Input: part model. Units: mm. Frame: model coordinates. A direction names the side the tool comes from. Coordinates: 2 decimals unless noted, no trailing zeros. Loops run counter-clockwise (first coordinate to the right, second up) from the corner with the lowest first, then second, coordinate; pieces in that order, holes last.
Item 1: Ray query, line 1 along Y through (x, z) = (43, 1.4) (3 decimals); line 2 along Y through (x, z) = (12.7, 1.1); line 3 along Y through (x, z) = (63.5, 0.8) (3 decimals). Return the intervals inside material, ascending.
Item 2: Contact query for flat-ended pins moving along their axis: P1, Ø1, axis at x = 19, z = 2, coming from the +Y side; P2, Ø1, axis at y = 23.5, z = 1, coming from the -X side; P3, Ø1, axis at y = -42, z = 2, coming from the -X side; P4, Ø8, axis at x = 77, y = -21, coming from the -Z side. Output: stop coordinate, or through.
Item 3: Section B-B on x = 44. Return loops of the section in (y, z) (3 decimals).
Item 4: Reachability of faces 4 (the flat face through (62, -53.975, 2)), 5 (the cylindrical face through (57.191, 5.716, 1.61)) from +Z, -Z, +X, -X, +Y, -Y: full face, straight path, thin tool, end or side. Return the list, or none.
Item 5: Section A-A on y = 38.1. Return loops of the section in (x, z) (3 decimals), and give its area (3 significant figures).
Item 6: Section D-D on y = 12.7. Return loops of the section in (x, z) (3 decimals).
Item 7: Section C-C on x = 34.5. Return loops of the section in (y, z) (3 decimals), and give its area (3 significant figures).
Item 8: Pull-direction query (Y, two-part tool) for faces 1 (the cylindrical face through (0.772, 25.036, 1.61)), 2 (the cylindrical face through (87.089, -52.065, 1.61)), 3 (the flat face through (25.4, 24, 2)); classes: released by +Y, released by -Y, zero draft, split by the parting line, or undercut.
```python
from build123d import *

# Parameters (mm, degrees)
SKETCH1_R           = 2.4892
BOSS_EXTRUDE1_DEPTH = 3.175
FILLET1_R           = 6.35
CUT_EXTRUDE1_DEPTH  = 105.050907012
FILLET3_R           = 3.175


with BuildPart() as part:
    # Sketch1 → Boss-Extrude1 (new body)
    with BuildSketch(Plane.XY):
        Polygon((0, 25.4), (38.1, 50.8), (88.9, 50.8), (88.9, -53.975), (38.1, -53.975), (0, 0), align=None)
        with Locations((12.7, 12.7)):
            Circle(SKETCH1_R, mode=Mode.SUBTRACT)
        with Locations((25.4, 12.7)):
            Circle(SKETCH1_R, mode=Mode.SUBTRACT)
        with Locations((50.8, 38.1)):
            Circle(SKETCH1_R, mode=Mode.SUBTRACT)
        with Locations((63.5, 38.1)):
            Circle(SKETCH1_R, mode=Mode.SUBTRACT)
        with Locations((76.2, 38.1)):
            Circle(SKETCH1_R, mode=Mode.SUBTRACT)
        with Locations((50.8, -41.275)):
            Circle(SKETCH1_R, mode=Mode.SUBTRACT)
        with Locations((76.2, -41.275)):
            Circle(SKETCH1_R, mode=Mode.SUBTRACT)
        with Locations((63.5, -41.275)):
            Circle(SKETCH1_R, mode=Mode.SUBTRACT)
    extrude(amount=BOSS_EXTRUDE1_DEPTH)

    # Fillet1
    fillet1_edges = [part.edges().sort_by_distance(p)[0] for p in [
        (0, 0, 1.5875),
        (0, 25.4, 1.5875),
        (38.1, 50.8, 1.5875),
        (88.9, 50.8, 1.5875),
        (88.9, -53.975, 1.5875),
        (38.1, -53.975, 1.5875),
    ]]
    fillet(fillet1_edges, radius=FILLET1_R)

    # Sketch2 → Cut-Extrude1 (cut, through all)
    with BuildSketch(Plane.XY):
        Polygon((25.4, -24.60625), (25.4, 6.35), (6.35, 6.35), align=None)
        Polygon((53.158456892, -1.5875), (31.75, 26.511099671), (31.75, 6.35), (31.75, -29.686099671), align=None)
        Polygon((78.558456892, -34.925), (57.15, -6.826400329), (35.741543108, -34.925), align=None)
        Polygon((82.55, 26.511099671), (61.141543108, -1.5875), (82.55, -29.686099671), align=None)
        Polygon((35.741543108, 31.75), (57.15, 3.651400329), (78.558456892, 31.75), align=None)
        Polygon((6.35, 19.05), (25.4, 19.05), (25.4, 31.75), align=None)
    extrude(amount=CUT_EXTRUDE1_DEPTH, mode=Mode.SUBTRACT)

    # Fillet3
    fillet3_edges = [part.edges().sort_by_distance(p)[0] for p in [
        (25.4, 31.75, 1.5875),
        (6.35, 19.05, 1.5875),
        (25.4, 19.05, 1.5875),
        (57.15, -6.826400329, 1.5875),
        (35.741543108, -34.925, 1.5875),
        (78.558456892, -34.925, 1.5875),
        (53.158456892, -1.5875, 1.5875),
        (31.75, 26.511099671, 1.5875),
        (31.75, -29.686099671, 1.5875),
        (78.558456892, 31.75, 1.5875),
        (35.741543108, 31.75, 1.5875),
        (57.15, 3.651400329, 1.5875),
        (82.55, -29.686099671, 1.5875),
        (82.55, 26.511099671, 1.5875),
        (61.141543108, -1.5875, 1.5875),
        (25.4, -24.60625, 1.5875),
        (25.4, 6.35, 1.5875),
        (6.35, 6.35, 1.5875),
    ]]
    fillet(fillet3_edges, radius=FILLET3_R)


solid = part.part
```
Results found:
1. line 1: y = -53.975 to -34.925, -25.398 to -14.92, 11.745 to 22.223, 31.75 to 50.8
1. line 2: y = -17.99 to -3.97, 6.35 to 10.21, 15.19 to 33.87
1. line 3: y = -53.975 to -43.764, -38.786 to -34.925, -15.161 to -4.683, 1.508 to 11.986, 31.75 to 35.611, 40.589 to 50.8
2. P1: stops at y = 38.4
2. P2: stops at x = 0.08
2. P3: stops at x = 29.29
2. P4: stops at z = 0
3. outline: (-53.975, 0) - (-34.925, 0) - (-34.925, 3.175) - (-53.975, 3.175) - close; (-24.086, 0) - (-13.608, 0) - (-13.608, 3.175) - (-24.086, 3.175) - close; (10.433, 0) - (20.911, 0) - (20.911, 3.175) - (10.433, 3.175) - close; (31.75, 0) - (50.8, 0) - (50.8, 3.175) - (31.75, 3.175) - close
4. face 4: +Z, -Z, +X, -X, -Y
4. face 5: +Z, -Z
5. outline: (19.05, 0) - (48.311, 0) - (48.311, 3.175) - (19.05, 3.175) - close; (53.289, 0) - (61.011, 0) - (61.011, 3.175) - (53.289, 3.175) - close; (65.989, 0) - (73.711, 0) - (73.711, 3.175) - (65.989, 3.175) - close; (78.689, 0) - (88.9, 0) - (88.9, 3.175) - (78.689, 3.175) - close
5. area: 174 mm2
6. outline: (0, 0) - (10.211, 0) - (10.211, 3.175) - (0, 3.175) - close; (15.189, 0) - (22.911, 0) - (22.911, 3.175) - (15.189, 3.175) - close; (27.889, 0) - (31.75, 0) - (31.75, 3.175) - (27.889, 3.175) - close; (42.273, 0) - (50.256, 0) - (50.256, 3.175) - (42.273, 3.175) - close; (64.044, 0) - (72.027, 0) - (72.027, 3.175) - (64.044, 3.175) - close; (82.55, 0) - (88.9, 0) - (88.9, 3.175) - (82.55, 3.175) - close
7. outline: (-48.875, 0) - (-23.426, 0) - (-23.426, 3.175) - (-48.875, 3.175) - close; (20.251, 0) - (48.4, 0) - (48.4, 3.175) - (20.251, 3.175) - close
7. area: 170 mm2
8. face 1: released by +Y
8. face 2: released by -Y
8. face 3: undercut
